Here's how the part is built. I have some questions about the finished solid (model axes, mm). Give positions to 0.01 mm unless a question says otherwise; leave off trailing zeros. Loops run counter-clockwise (first coordinate to the right, second up) from the corner with the lowest first, then second, coordinate; pieces in that order, holes last. Notation, with made-up numbers: (16, 71.25) - (39, 71.25) arc R9 ccw to (39, 88.25) - close; hole circle Ø5 at (-2, 48). An arc over 180 degrees is marked (long way). Return JSON: item names as keys, results as strings. Group by question number.
(1) If we section it at B-B (z = 7): Please give me the cut outline in (x, y), then the cut area to 3 significant figures.
(2) I need wall thicknesses on probe 1 along Y at (x, z) = (0.5, 3.75); probe 2 along X at (y, z) = (2.25, 5.25); probe 3 along X at (y, z) = (0.75, 6). Which ranges of each line are inside material? Lowest first, please. Write a range as [from, to].
(3) If we section it at D-D (y = -7.5): Please give me the cut outline in (x, z).
(4) For P1, Ø2, axis at y = 4, z = 3, coming from the +X side; P2, Ø3, axis at y = -4.5, z = 6, coming from the +X side; P3, Ø1.5, axis at y = -2, z = 3.5, coming from the +X side, each with a flat end and sliding along its axis, tell me the tip position at first contact or that it passes through.
(5) If we mould it in two halves opening along X, with no side actions, what happens to faces 1 (the cylindrical face through (-2.285, 3.584, 4.93)), 2 (the flat face through (-7.553, -4.009, 9.442)), 3 (the flat face through (7.54, 4, 9.46))? For each: released by +X, released by -X, zero draft, split by the parting line, or undercut.
(6) If we section it at A-A (y = 1.75): Please give me the cut outline in (x, z), then the cut area to 3 significant figures.
(7) If we section it at C-C (x = 0): Please give me the cut outline in (y, z).
```python
from build123d import *

# Parameters (mm, degrees)
F1_DEPTH = 10
F3_D     = 8.5
F4_SIZE  = 1.1


with BuildPart() as f1:
    # F0 (on Top) → F1 (new body)
    with BuildSketch(Plane.XY):
        Polygon((10.4961740703, -0.2834252726), (5.4935405213, 8.9482407512), (-5.0026335491, 9.2316660237), (-10.4961740703, 0.2834252726), (-5.4935405213, -8.9482407512), (5.0026335491, -9.2316660237), align=None)
    extrude(amount=F1_DEPTH)

    # F3 (through all)
    with Locations(Plane.XY.offset(10)):
        with Locations((0, 0)):
            Hole(F3_D / 2)

    # F4
    f4_edges = [f1.edges().sort_by_distance(p)[0] for p in [
        (-7.994857, -4.332408, 10),
        (-7.749404, 4.757546, 10),
        (0.245453, 9.089953, 10),
        (7.994857, 4.332408, 10),
        (7.749404, -4.757546, 10),
        (-0.245453, -9.089953, 10),
        (-0.245453, -9.089953, 0),
        (7.749404, -4.757546, 0),
        (7.994857, 4.332408, 0),
        (0.245453, 9.089953, 0),
        (-7.749404, 4.757546, 0),
        (-7.994857, -4.332408, 0),
    ]]
    chamfer(f4_edges, length=F4_SIZE)


solid = f1.part
```
Values:
{
 "1": {"outline": "(-10.5, 0.28) - (-5.49, -8.95) - (5, -9.23) - (10.5, -0.28) - (5.49, 8.95) - (-5, 9.23) - close; hole circle Ø8.5 at (0, 0)", "area": "230 mm2"},
 "2": {"probe 1": "[-9.11, -4.22], [4.22, 9.08]", "probe 2": "[-9.29, -3.61], [3.61, 9.12]", "probe 3": "[-10.21, -4.18], [4.18, 9.94]"},
 "3": {"outline": "(-6.28, 1.1) - (-5.03, 0) - (4.77, 0) - (6.07, 1.1) - (6.07, 8.9) - (4.77, 10) - (-5.03, 10) - (-6.28, 8.9) - close"},
 "4": {"P1": "x = 8.72", "P2": "x = 8.83", "P3": "x = 9.9"},
 "5": {"face 1": "undercut", "face 2": "released by -X", "face 3": "released by +X"},
 "6": {"outline": "(-9.6, 1.1) - (-8.31, 0) - (-3.87, 0) - (-3.87, 10) - (-8.31, 10) - (-9.6, 8.9) - close; (3.87, 0) - (8.14, 0) - (9.39, 1.1) - (9.39, 8.9) - (8.14, 10) - (3.87, 10) - close", "area": "110 mm2"},
 "7": {"outline": "(-9.1, 1.1) - (-8, 0) - (-4.25, 0) - (-4.25, 10) - (-8, 10) - (-9.1, 8.9) - close; (4.25, 0) - (8, 0) - (9.1, 1.1) - (9.1, 8.9) - (8, 10) - (4.25, 10) - close"}
}
